Can you work these out from the model? Positions are in its coordinate system, mm. A direction names the side the tool comes from. Coordinates: 2 decimals unless noted, no trailing zeros. Order: outer loops, then holes, each group sorted by start corner. A loop starts at its lowest first (then second) coordinate and runs counter-clockwise, first axis right, second up. Notation, with made-up numbers: (-15, 35) -> (22, 35) arc R27 ccw to (22, 63) -> close; hole circle Ø2 at (18, 82.5). An arc over 180 degrees is marked (long way). Answer in a Markdown table with one row per item. Add a question column.
1. Imagine slicing it at B-B on y = 14.5. Write out the boundary of the cut face in (x, z), plus the area to 3 significant figures.
2. If I drill on line 1 along Y through (x, z) = (11.95, 9.45); line 2 along X through (y, z) = (16, 3.25); line 3 along Y through (x, z) = (-6, 7), over which ranges is the centre line in solid material (lowest first)? Write a range as [from, to].
3. On a 3-axis mill with a long thin cutter (end or side, diameter ignored), from which of +Z, -Z, +X, -X, +Y, -Y can I reach the whole of each face in a straight line? I mean faces 4 (the face through (-24, 14.4, 4.8)), 5 (the face through (-6.692, -21.865, 3.944)), 6 (the face through (24.9, -13.7, 5.9)). Say none if no direction works.
4. Will these pins go through, and if not, where does the flat tip stop? pin 1 (2.5 mm diameter, centred on x = 11, y = -23.5, fed in from -Z); pin 2 (1.8 mm diameter, centred on y = -24, z = 3.5, fed in from -X); pin 3 (5 mm diameter, centred on x = 12.5, z = 1, fed in from -Y).
5. We'd pull the mould along X, two halves only. Please class faces 1 (the face through (0, 25, 6)), 2 (the face through (8.528, -11.287, 3.944)), 3 (the face through (-32.25, 0, 6)): pulls with the +X half, pulls with the -X half, needs draft (parallel to the pull), parting line crosses it, or undercut.
6. Imagine slicing it at A-A on x = -25. Write out the boundary of the cut face in (y, z), plus the area to 3 significant figures.
7. Imagine slicing it at D-D on x = -4.5. Write out the boundary of the cut face in (y, z).
from build123d import *

# Parameters (mm, degrees)
F0_W           = 64.5
F0_H           = 50
F1_DEPTH       = 10
F3_DEPTH       = 8
F4_R           = 4
F5_DEPTH       = 25
F6_R           = 4.1
F7_DEPTH       = 23
F8_R           = 5
F9_DEPTH       = 64.501
F10_R          = 7.234183596
F11_DEPTH      = 24
F11_DEPTH_BACK = 25
F12_R          = 2
F13_W          = 7.2386283427
F13_H          = 5.7293735445
F14_DEPTH      = 25


with BuildPart() as f1:
    # F0 (on Top) → F1 (new body)
    with BuildSketch(Plane.XY):
        Rectangle(F0_W, F0_H)
    extrude(amount=F1_DEPTH)

    # F2 (on face) → F3 (cut)
    with BuildSketch(Plane(origin=(0, 0, 0), x_dir=(1, 0, 0), z_dir=(0, 0, -1))):
        Polygon((-5.2, 13.2086570489), (-5.2, 21.002885683), (-11.95, 24.9), (-18.7, 21.002885683), (-18.7, 13.2086570489), (-11.95, 9.3115427319), align=None)
        Polygon((18.7, 21.002885683), (11.95, 24.9), (5.2, 21.002885683), (5.2, 13.2086570489), (11.95, 9.3115427319), (18.7, 13.2086570489), align=None)
    extrude(amount=-F3_DEPTH, mode=Mode.SUBTRACT)

    # F4 (on face) → F5 (cut)
    with BuildSketch(Plane(origin=(0, 0, 8), x_dir=(1, 0, 0), z_dir=(0, 0, -1))):
        with Locations((-11.95, 17.1057713659)):
            Circle(F4_R)
        with Locations((11.95, 17.1057713659)):
            Circle(F4_R)
    extrude(amount=-F5_DEPTH, mode=Mode.SUBTRACT)

    # F6 (on face) → F7 (cut)
    with BuildSketch(Plane.XZ.offset(25)):
        with Locations((25, 10)):
            Circle(F6_R)
        with Locations((-25, 10)):
            Circle(F6_R)
    extrude(amount=-F7_DEPTH, mode=Mode.SUBTRACT)

    # F8 (on face) → F9 (cut, through all)
    with BuildSketch(Plane.YZ.offset(32.25)):
        with Locations((14.5, 10)):
            Circle(F8_R)
    extrude(amount=-F9_DEPTH, mode=Mode.SUBTRACT)

    # F10 (on Right) → F11 (cut, two sides)
    with BuildSketch(Plane.YZ) as f11_sk:
        with Locations((14.5, 10)):
            Circle(F10_R)
    extrude(amount=-F11_DEPTH, mode=Mode.SUBTRACT)
    extrude(f11_sk.sketch, amount=F11_DEPTH_BACK, mode=Mode.SUBTRACT)

    # F12
    f12_edges = [f1.edges().sort_by_distance(p)[0] for p in [
        (0, 25, 0),
        (32.25, 0, 0),
        (-32.25, 0, 0),
        (32.25, 25, 5),
        (-32.25, 25, 5),
        (-32.25, -25, 5),
        (32.25, -25, 5),
    ]]
    fillet(f12_edges, radius=F12_R)

    # F13 (on face) → F14 (cut)
    with BuildSketch(Plane(origin=(0, 0, 8), x_dir=(1, 0, 0), z_dir=(0, 0, -1))):
        with Locations((-11.8464780971, 24.8996280134)):
            Rectangle(F13_W, F13_H)
        Polygon((15.4657922685, 27.7643147856), (8.2271639258, 27.7643147856), (8.2271639258, 22.7506195904), (11.95, 24.9), (15.4657922685, 22.8701563874), align=None)
    extrude(amount=F14_DEPTH, mode=Mode.SUBTRACT)


solid = f1.part
Answers follow:
| question | item | result |
|---|---|---|
| 1 | outline | (-32.25, 2) arc R2 ccw to (-30.25, 0) -> (30.25, 0) arc R2 ccw to (32.25, 2) -> (32.25, 5) -> (25, 5) -> (25, 2.77) -> (-24, 2.77) -> (-24, 5) -> (-32.25, 5) -> close |
| 1 | area | 211 mm² |
| 2 | line 1 | y = [-25, -21.11], [-13.11, 7.29], [21.71, 25] |
| 2 | line 2 | x = [-32.25, -24], [25, 32.25] |
| 2 | line 3 | y = [-25, -21.46], [-12.75, 7.92], [21.08, 25] |
| 3 | face 4 | +Z |
| 3 | face 5 | -Z |
| 3 | face 6 | +Z, -Y |
| 4 | pin 1 | stops at z = 8 |
| 4 | pin 2 | stops at x = -32.25 |
| 4 | pin 3 | stops at y = -11.07 |
| 5 | face 1 | needs draft |
| 5 | face 2 | undercut |
| 5 | face 3 | pulls with the -X half |
| 6 | outline | (-25, 0) -> (23, 0) arc R2 ccw to (25, 2) -> (25, 10) -> (19.5, 10) arc R5 cw to (9.5, 10) -> (-2, 10) -> (-2, 5.9) -> (-25, 5.9) -> close |
| 6 | area | 366 mm² |
| 7 | outline | (-25, 0) -> (23, 0) arc R2 ccw to (25, 2) -> (25, 10) -> (21.73, 10) arc R7.23 cw to (7.27, 10) -> (-25, 10) -> close |
